The listing builds one solid part. Answer for the finished solid, in the listing's coordinates (mm). A direction names the side the tool comes from. Round coordinates to 2 decimals unless told otherwise and drop trailing zeros. Loops run counter-clockwise (first coordinate to the right, second up) from the corner with the lowest first, then second, coordinate; pieces in that order, holes last. Notation, with made-up numbers: M 18.25,67 L 65.25,67 A20 cw 65.25,86 Z; hole C 48,87.5 d3. An arc over 180 degrees is marked long. Answer as a JSON object with one key per item and string values.
Autodesk Inventor part; units mm, degrees
ref_plane "dia1_XY" through (0, 2.3749, 0) normal (1, 0, 0) x (0, 0, -1)
ref_plane "dia1_YZ" through (0, 2.3749, 0) normal (0, 0, -1) x (0, 1, 0)
ref_plane "dia1_ZX" through (0, 2.3749, 0) normal (0, 1, 0) x (1, 0, 0)
sketch "Sketch_1" plane through (0, 0, 0) normal (0, 0, 1) x (1, 0, 0)
  line L0 (283.2608, 0) -> (0, 0)
  line L1 (0, 0) -> (0, 2.3749)
  line L2 (0, 2.3749) -> (157.1752, 2.3749)
  line L3 (157.1752, 2.3749) -> (157.1752, 5.6197)
  line L4 (157.1752, 5.6197) -> (283.2608, 5.6197)
  line L5 (283.2608, 5.6197) -> (283.2608, 0)
  line L6 (283.2608, 0) -> (0, 0)
revolve "Revolution1" add sketch "Sketch_1" angle 360 about axis through (283.2608, 0, 0) along (1, 0, 0)
sketch "Sketch_3" plane through (0, 0, 0) normal (0, 0, 1) x (1, 0, 0)
  line L0 (0, 0) -> (-12.7, 0)
  line L1 (-12.7, 0) -> (-12.7, 1.9406)
  line L2 (-12.7, 1.9406) -> (-12.2276, 2.413)
  line L3 (-12.2276, 2.413) -> (0, 2.413)
  line L4 (0, 2.413) -> (0, 0)
  line L5 (0, 0) -> (-12.7, 0)
revolve "Revolution2" add sketch "Sketch_3" angle 360 about axis through (0, 0, 0) along (1, 0, 0)
thread "Thread1"
sketch "Sketch_30" plane through (0, 0, 0) normal (0, 0, 1) x (1, 0, 0)
  line L0 (0, 0) -> (-0.254, 0)
  line L1 (-0.254, 2.159) -> (0, 2.159)
  line L2 (0, 2.159) -> (0, 2.667)
  line L3 (0, 2.667) -> (-0.254, 2.667)
  line L4 (-0.254, 2.667) -> (-0.254, 2.159)
revolve "Revolution3" cut sketch "Sketch_30" angle 360 about axis through (0, 0, 0) along (1, 0, 0)
ref_plane "dia1_XY" through (0, 2.3749, 0) normal (1, 0, 0) x (0, 0, -1)
ref_plane "dia1_YZ" through (0, 2.3749, 0) normal (0, 0, -1) x (0, 1, 0)
ref_plane "dia1_ZX" through (0, 2.3749, 0) normal (0, 1, 0) x (1, 0, 0)
ref_plane "dia12_XY" through (0, 0, 6.1468) normal (1, 0, 0) x (0, 0, -1)
ref_plane "dia12_YZ" through (0, 0, 6.1468) normal (0, 0, -1) x (0, 1, 0)
ref_plane "dia12_ZX" through (0, 0, 6.1468) normal (0, 1, 0) x (1, 0, 0)
ref_plane "dia1r_XY" through (0, 0, 9.3726) normal (1, 0, 0) x (0, 0, -1)
ref_plane "dia1r_YZ" through (0, 0, 9.3726) normal (0, 0, -1) x (0, 1, 0)
ref_plane "dia1r_ZX" through (0, 0, 9.3726) normal (0, 1, 0) x (1, 0, 0)
ref_plane "dia2_XY" through (0, -2.3749, 0) normal (1, 0, 0) x (0, 0, -1)
ref_plane "dia2_YZ" through (0, -2.3749, 0) normal (0, 0, -1) x (0, 1, 0)
ref_plane "dia2_ZX" through (0, -2.3749, 0) normal (0, 1, 0) x (1, 0, 0)
ref_plane "dia22_XY" through (0, 0, -6.1468) normal (1, 0, 0) x (0, 0, -1)
ref_plane "dia22_YZ" through (0, 0, -6.1468) normal (0, 0, -1) x (0, 1, 0)
ref_plane "dia22_ZX" through (0, 0, -6.1468) normal (0, 1, 0) x (1, 0, 0)
ref_plane "dia2r_XY" through (0, 0, -9.3726) normal (1, 0, 0) x (0, 0, -1)
ref_plane "dia2r_YZ" through (0, 0, -9.3726) normal (0, 0, -1) x (0, 1, 0)
ref_plane "dia2r_ZX" through (0, 0, -9.3726) normal (0, 1, 0) x (1, 0, 0)
ref_plane "rl1_XY" through (-12.7, 0, 0) normal (1, 0, 0) x (0, 0, -1)
ref_plane "rl1_YZ" through (-12.7, 0, 0) normal (0, 0, -1) x (0, 1, 0)
ref_plane "rl1_ZX" through (-12.7, 0, 0) normal (0, 1, 0) x (1, 0, 0)
ref_plane "rl2_XY" through (0, 0, 0) normal (1, 0, 0) x (0, 0, -1)
ref_plane "rl2_YZ" through (0, 0, 0) normal (0, 0, -1) x (0, 1, 0)
ref_plane "rl2_ZX" through (0, 0, 0) normal (0, 1, 0) x (1, 0, 0)
ref_plane "rod_cp_XY" through (0, 0, 0) normal (1, 0, 0) x (0, 0, -1)
ref_plane "rod_cp_YZ" through (0, 0, 0) normal (0, 0, -1) x (0, 1, 0)
ref_plane "rod_cp_ZX" through (0, 0, 0) normal (0, 1, 0) x (1, 0, 0)
ref_plane "thd1_XY" through (-12.7, 2.413, 0) normal (1, 0, 0) x (0, 0, -1)
ref_plane "thd1_YZ" through (-12.7, 2.413, 0) normal (0, 0, -1) x (0, 1, 0)
ref_plane "thd1_ZX" through (-12.7, 2.413, 0) normal (0, 1, 0) x (1, 0, 0)
ref_plane "thd2_XY" through (-12.7, -2.413, 0) normal (1, 0, 0) x (0, 0, -1)
ref_plane "thd2_YZ" through (-12.7, -2.413, 0) normal (0, 0, -1) x (0, 1, 0)
ref_plane "thd2_ZX" through (-12.7, -2.413, 0) normal (0, 1, 0) x (1, 0, 0)
ref_plane "to_rod_clevis_XY" through (-12.7, 0, 0) normal (1, 0, 0) x (0, 0, -1)
ref_plane "to_rod_clevis_YZ" through (-12.7, 0, 0) normal (0, 0, -1) x (0, 1, 0)
ref_plane "to_rod_clevis_ZX" through (-12.7, 0, 0) normal (0, 1, 0) x (1, 0, 0)
properties part number "015.5-P0000_rod"
Item 1: Flat-ended cylindrical pins translate along their axes: P1, Ø3, axis at x = 219.5, y = 3, coming from the +Z side; P2, Ø5, axis at x = 35.5, z = -3.5, coming from the -Y side; P3, Ø3, axis at x = 185, z = 2.5, coming from the -Y side. Find the tip coordinate at first contact, or state that the pin passes through.
Values follow:
{"P1": "z = 5.42", "P2": "y = -2.15", "P3": "y = -5.53"}
Item 2: Straight lines are drawn through the part: line 1 (X direction, y = 2.25, z = -4.5); line 2 (Y direction, x = 234, z = -0.75); line 3 (X direction, y = 1.25, z = 1.5). For each, find the intervals that lie inside material, in ascending order.
Values follow:
{"line 1": "157.18 to 283.26", "line 2": "-5.57 to 5.57", "line 3": "-12.69 to 283.26"}
Item 3: The part is cut by section C-C (x = 81). Give the vertices of the cut face in (y, z).
Values follow:
{"outline": "C 0,0 d4.75"}
Item 4: The part is cut by section A-A (z = 0). Give the vertices of the cut face in (x, y).
Values follow:
{"outline": "M -12.7,-1.94 L -12.23,-2.41 L -0.25,-2.41 L -0.25,-2.16 L 0,-2.16 L 0,-2.37 L 157.18,-2.37 L 157.18,-5.62 L 283.26,-5.62 L 283.26,5.62 L 157.18,5.62 L 157.18,2.37 L 0,2.37 L 0,2.16 L -0.25,2.16 L -0.25,2.41 L -12.23,2.41 L -12.7,1.94 Z"}
Item 5: The part is cut by section B-B (x = 237.5). Give the vertices of the cut face in (y, z), then the cut area to 3 significant figures.
Values follow:
{"outline": "C 0,0 d11.24", "area": "99.2 mm^2"}
Item 6: Which of the six approach directions +Z, -Z, +X, -X, +Y, -Y give full straight-line access (tool end or side, diameter ignored) to faces 1 (the face through (-6.157, -1.915, -1.468)), 2 (the face through (221.101, -1.218, -5.486))?
Values follow:
{"face 1": "-X", "face 2": "+X, -X"}
